Part model, mm, in its own coordinate system. A direction names the side the tool comes from. Give positions to 0.01 mm unless a question says otherwise; leave off trailing zeros. Order: outer loops, then holes, each group sorted by start corner. A loop starts at its lowest first (then second) coordinate and runs counter-clockwise, first axis right, second up. Notation, with made-up numbers: (45.5, 59) - (68.5, 59) arc R13 ccw to (68.5, 75) - close; hole circle Ø6 at (40.5, -20.75). An arc over 180 degrees is marked (long way). One line per item, written item: value.
```python
from build123d import *

# Parameters (mm, degrees)
SKETCH1_R           = 23
BOSS_EXTRUDE1_DEPTH = 12
SKETCH2_R           = 15
BOSS_EXTRUDE2_DEPTH = 180
SCALE1_SCALE        = 0.33


with BuildPart() as part:
    # Sketch1 → Boss-Extrude1 (new body)
    with BuildSketch(Plane(origin=(0, 0, 0), x_dir=(1, 0, 0), z_dir=(0, 1, 0))):
        with Locations(Location((0, 0, 0), (0, 0, 270))):
            Circle(SKETCH1_R)
    extrude(amount=BOSS_EXTRUDE1_DEPTH)

    # Sketch2 → Boss-Extrude2 (add)
    with BuildSketch(Plane(origin=(0, 12, 0), x_dir=(1, 0, 0), z_dir=(0, 1, 0))):
        with Locations(Location((0, 0, 0), (0, 0, 90))):
            Circle(SKETCH2_R)
    extrude(amount=BOSS_EXTRUDE2_DEPTH)

    # Sketch4 → Cut-Revolve4 (revolve, cut)
    with BuildSketch(Plane(origin=(0, 180, 0), x_dir=(1, 0, 0), z_dir=(0, 1, 0)), mode=Mode.PRIVATE) as cut_revolve4_sk:
        Polygon((30, 0), (-30, 0), (-30, 3), (30, 2.5), align=None)
    revolve(cut_revolve4_sk.sketch.rotate(Axis((30, 180, 0), (-1, 0, 0)), 43.222244731), axis=Axis((30, 180, 0), (-1, 0, 0)), mode=Mode.SUBTRACT)


with BuildPart() as part_1:
    # Scale1: scaled about (0.002156462, 88.550518563, 3e-09)
    add(part.part.scale(SCALE1_SCALE).moved(Location((0.00144483, 59.328847437, 2e-09))))


solid = part_1.part
```
1) Slice it at D-D on x = -5.5. Write the cut outline in (y, z).
Answer:
outline: (59.33, -5.23) - (63.29, -5.23) - (63.29, 5.23) - (59.33, 5.23) - close
2) Slice it at A-A on x = 2.75. Write the cut outline in (y, z), then the cut area to 3 significant figures.
Answer:
outline: (59.33, -7.07) - (63.29, -7.07) - (63.29, -4.12) - (122.69, -4.12) - (122.69, 4.12) - (63.29, 4.12) - (63.29, 7.07) - (59.33, 7.07) - close; hole circle Ø1.77 at (118.73, 0)
area: 543 mm2
3) Slice it at C-C on y = 81.5. Write the cut outline in (x, z), then the cut area to 3 significant figures.
Answer:
outline: circle Ø9.9 at (0, 0)
area: 77.0 mm2
4) Two-plate mould, pull along Z, no slides. Class faces 1 (the face through (-5, 63.289, 2)), 2 (the face through (0.07, 117.84, 0.17)), 3 (the face through (-7.408, 61.281, -1.645)): pulls with the +Z half, pulls with the -Z half, needs draft (parallel to the pull), parting line crosses it, or undercut.
Answer:
face 1: needs draft
face 2: undercut
face 3: parting line crosses it
5) Wall check: line 1 along X through (y, z) = (100.5, -0.25); line 2 along Y through (x, z) = (4, 0); line 3 along X through (y, z) = (95, 0). Give the ranges that are in metal, low to high. Write a range as [from, to].
Answer:
line 1: x = [-4.94, 4.95]
line 2: y = [59.33, 117.85], [119.6, 122.69]
line 3: x = [-4.95, 4.95]
6) Which spindle directions (+Z, -Z, +X, -X, +Y, -Y) get a long thin tool onto all of the face, cutting with end or side? Do faces 4 (the face through (0, 122.689, 0)), 5 (the face through (4.834, 92.573, 1.073)). Say none if no direction does.
Answer:
face 4: +Z, -Z, +X, -X, +Y
face 5: +Y
7) Slice it at B-B on z = -3.75. Write the cut outline in (x, y), then the cut area to 3 significant figures.
Answer:
outline: (-6.6, 59.33) - (6.6, 59.33) - (6.6, 63.29) - (3.23, 63.29) - (3.23, 122.69) - (-3.23, 122.69) - (-3.23, 63.29) - (-6.6, 63.29) - close
area: 436 mm2
8) Drop flat-ended pins along their axis: P1, Ø1.5, axis at y = 67, z = 4.5, coming from the +X side; P2, Ø8, axis at x = 4, y = 80.5, coming from the -Z side; P3, Ø3, axis at y = 115.5, z = -1, coming from the +X side. Give the stop position or say it passes through.
Answer:
P1: stops at x = 3.23
P2: stops at z = -4.95
P3: stops at x = 4.95
